Design review of the part built by this model. Coordinates are the model's own, in mm. A direction names the side the tool comes from. Round coordinates to 2 decimals unless told otherwise and drop trailing zeros. Write each loop counter-clockwise with the first axis right and the second up, starting at its lowest first coordinate (ties: lowest second). Pieces come first, ordered by that corner, then holes. Notation, with made-up numbers: (-8, -14.5) -> (17, -14.5) arc R8 ccw to (17, -4.5) -> close; hole circle Ø3 at (31.25, 40). An arc over 180 degrees is marked (long way). Write item = value, one per line. Start each with the question number.
Item 1: To check wall thickness, follow L1, parallel to Z at x = 71.5, y = 1.75; L2, parallel to X at y = 4.5, z = -40 (3 decimals); L3, parallel to Z at x = -37.5, y = 1.75. State the ranges of each line that lie inside material, in increasing order.
Item 2: Add section B-B, the plane z = -7.5. State the section outline as (x, y) points (3 decimals).
Item 3: Add section A-A, the plane z = -58. State the section outline as (x, y) points (3 decimals), then the cut area to 3 significant figures.
Item 4: Machinability: for faces 1 (the flat face through (-2, 3, -76.2)), 2 (the flat face through (117.475, 3, 67)), which of the approach directions +Z, -Z, +X, -X, +Y, -Y give a long, thin tool a straight path to every point of the face, cutting with its end or side? Answer none if there is none.
Item 5: Add section D-D, the plane y = 4. State how many separate pieces and enclosed holes the cut face has, then the cut area to 3 significant figures.
Item 6: Add section C-C, the plane x = 76. State the section outline as (y, z) points.
Item 7: Mouldability with a two-part tool opening along X and no side actions: class faces 3 (the flat face through (26, 0, -1)), 4 (the flat face through (-59, 3, -63.505)), 5 (the flat face through (127, 3, 1)) as released by +X, released by -X, zero draft, split by the parting line, or undercut.
from build123d import *

# Parameters (mm, degrees)
SKETCH1_W           = 254
SKETCH1_H           = 152.4
SKETCH1_W_2         = 6.35
SKETCH1_H_2         = 101.6
SKETCH1_H_3         = 139.7
SKETCH1_W_3         = 98.425
SKETCH1_H_4         = 6.34492
SKETCH1_W_4         = 3.175
BOSS_EXTRUDE1_DEPTH = 6.35


with BuildPart() as part:
    # Sketch1 → Boss-Extrude1 (new body)
    with BuildSketch(Plane(origin=(0, 0, 0), x_dir=(1, 0, 0), z_dir=(0, 1, 0))):
        Rectangle(SKETCH1_W, SKETCH1_H)
        with Locations((117.475, 0)):
            Rectangle(SKETCH1_W_2, SKETCH1_H_2, mode=Mode.SUBTRACT)
        Rectangle(SKETCH1_W_2, SKETCH1_H_3, mode=Mode.SUBTRACT)
        with Locations((-117.475, 0)):
            Rectangle(SKETCH1_W_2, SKETCH1_H_2, mode=Mode.SUBTRACT)
        with Locations((-58.7375, 66.67754)):
            Rectangle(SKETCH1_W_3, SKETCH1_H_4, mode=Mode.SUBTRACT)
        with Locations((58.7375, -66.68262)):
            Rectangle(SKETCH1_W_3, SKETCH1_H_4, mode=Mode.SUBTRACT)
        with Locations((58.7375, 66.67754)):
            Rectangle(SKETCH1_W_3, SKETCH1_H_4, mode=Mode.SUBTRACT)
        with Locations((-58.7375, -66.67754)):
            Rectangle(SKETCH1_W_3, SKETCH1_H_4, mode=Mode.SUBTRACT)
        with Locations((-119.0625, -66.67754)):
            Rectangle(SKETCH1_W_4, SKETCH1_H_4, mode=Mode.SUBTRACT)
        with Locations((119.0625, -66.67754)):
            Rectangle(SKETCH1_W_4, SKETCH1_H_4, mode=Mode.SUBTRACT)
        with Locations((-119.0625, 66.67754)):
            Rectangle(SKETCH1_W_4, SKETCH1_H_4, mode=Mode.SUBTRACT)
        with Locations((119.0625, 66.67754)):
            Rectangle(SKETCH1_W_4, SKETCH1_H_4, mode=Mode.SUBTRACT)
    extrude(amount=BOSS_EXTRUDE1_DEPTH)


solid = part.part
Result set:
q1.L1 = -76.2 to -69.85, -63.51 to 63.51, 69.86 to 76.2
q1.L2 = -127 to -120.65, -114.3 to -3.175, 3.175 to 114.3, 120.65 to 127
q1.L3 = -76.2 to -69.85, -63.51 to 63.51, 69.85 to 76.2
q2.outline = (-127, 0) -> (-120.65, 0) -> (-120.65, 6.35) -> (-127, 6.35) -> close; (-114.3, 0) -> (-3.175, 0) -> (-3.175, 6.35) -> (-114.3, 6.35) -> close; (3.175, 0) -> (114.3, 0) -> (114.3, 6.35) -> (3.175, 6.35) -> close; (120.65, 0) -> (127, 0) -> (127, 6.35) -> (120.65, 6.35) -> close
q3.outline = (-127, 0) -> (-3.175, 0) -> (-3.175, 6.35) -> (-127, 6.35) -> close; (3.175, 0) -> (127, 0) -> (127, 6.35) -> (3.175, 6.35) -> close
q3.area = 1,570 mm²
q4.face_1 = -Z, +X, -X, +Y, -Y
q4.face_2 = +Y, -Y
q5.separate_pieces = 1
q5.enclosed_holes = 11
q5.area = 34,000 mm²
q6.outline = (0, -76.2) -> (6.35, -76.2) -> (6.35, -69.85) -> (0, -69.85) -> close; (0, -63.51) -> (6.35, -63.51) -> (6.35, 63.51) -> (0, 63.51) -> close; (0, 69.86) -> (6.35, 69.86) -> (6.35, 76.2) -> (0, 76.2) -> close
q7.face_3 = zero draft
q7.face_4 = undercut
q7.face_5 = released by +X
